Autodesk Inventor part; units mm, degrees
ref_plane "YZ Plane" through (0, 0, 0) normal (1, 0, 0) x (0, 1, 0)
ref_plane "XZ Plane" through (0, 0, 0) normal (0, 1, 0) x (-1, 0, 0)
ref_plane "XY Plane" through (0, 0, 0) normal (0, 0, 1) x (1, 0, 0)
sketch "Sketch1" plane through (0, 0, 0) normal (0, 0, 1) x (1, 0, 0)
  line L0 (3.6662, 6.35) -> (7.3323, 0)
  line L1 (7.3323, 0) -> (3.6662, -6.35)
  line L2 (3.6662, -6.35) -> (-3.6662, -6.35)
  line L3 (-3.6662, -6.35) -> (-7.3323, 0)
  line L4 (-7.3323, 0) -> (-3.6662, 6.35)
  line L5 (-3.6662, 6.35) -> (3.6662, 6.35)
  point P0 (0, 0)
  point P1 (0, 0)
  dimension "d0" = 12.7
extrude "Extrusion1" add sketch "Sketch1" along normal blind 82.55
sketch "Sketch3" plane through (0, 0, 82.55) normal (0, 0, 1) x (1, 0, 0)
  circle A0 centre (0, 0) radius 3.175
  dimension "d4" = 6.35
extrude "Extrusion2" cut sketch "Sketch3" against normal blind 25.4
sketch "Sketch4" plane through (0, 0, 0) normal (0, 0, -1) x (-1, 0, 0)
  circle A0 centre (0, 0) radius 3.175
  dimension "d7" = 6.35
extrude "Extrusion3" cut sketch "Sketch4" against normal blind 25.4
properties part number "WheelAxle" material "Aluminum-6061"
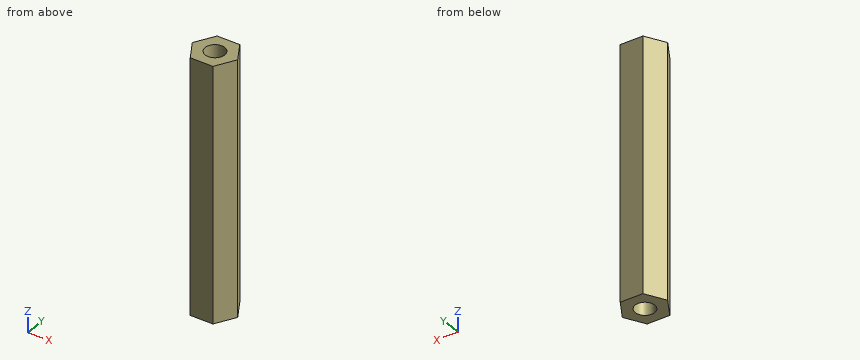
Source: CAD feature listing. Evaluate the final solid. Frame: model axes, mm. Give positions to 0.01 mm unless a question says otherwise; leave off trailing zeros. Write each loop counter-clockwise with the first axis right and the second up, starting at its lowest first coordinate (ties: lowest second). Pieces come first, ordered by that corner, then holes. Notation, with made-up numbers: (10.25, 73) -> (24.25, 73) arc R9 ccw to (24.25, 79) -> close; hole circle Ø8 at (-9, -36.75). An arc over 180 degrees is marked (long way). Return JSON: item names as keys, results as strings. Group by question number.
1. Section A-A, the plane z = 75.5. Output: boundary loops of the cut face in (x, y) (3 decimals).
2. Pin query (flat end, axial travel): pin 1 Ø3 at (x, y) = (-0.5, -0.5) entering from +Z; pin 2 Ø4 at (x, y) = (0, 0) entering from -Z; pin 3 Ø3 at (y, z) = (5, 23.5) entering from -X. Return the tip coordinate at first contact, or that it passes through.
3. Material intervals for line 1 (Y direction, x = 0, z = 73) (3 decimals); line 2 (Y direction, x = -2.5, z = 70.5); line 3 (X direction, y = 1.5, z = 24), sorted ascending. Write a range as from..to.
4. Section C-C, the plane z = 55. Output: boundary loops of the cut face in (x, y).
5. Section B-B, the plane x = 0. Output: boundary loops of the cut face in (y, z) (3 decimals).
6. Section D-D, the plane x = 5.25. Output: boundary loops of the cut face in (y, z), then the cut area to 3 significant figures.
Determined:
{
 "1": {"outline": "(-7.332, 0) -> (-3.666, -6.35) -> (3.666, -6.35) -> (7.332, 0) -> (3.666, 6.35) -> (-3.666, 6.35) -> close; hole circle Ø6.35 at (0, 0)"},
 "2": {"pin 1": "stops at z = 57.15", "pin 2": "stops at z = 25.4", "pin 3": "stops at x = -5.31"},
 "3": {"line 1": "y = -6.35..-3.175, 3.175..6.35", "line 2": "y = -6.35..-1.96, 1.96..6.35", "line 3": "x = -6.47..-2.8, 2.8..6.47"},
 "4": {"outline": "(-7.33, 0) -> (-3.67, -6.35) -> (3.67, -6.35) -> (7.33, 0) -> (3.67, 6.35) -> (-3.67, 6.35) -> close"},
 "5": {"outline": "(-6.35, 0) -> (-3.175, 0) -> (-3.175, 25.4) -> (3.175, 25.4) -> (3.175, 0) -> (6.35, 0) -> (6.35, 82.55) -> (3.175, 82.55) -> (3.175, 57.15) -> (-3.175, 57.15) -> (-3.175, 82.55) -> (-6.35, 82.55) -> close"},
 "6": {"outline": "(-3.61, 0) -> (3.61, 0) -> (3.61, 82.55) -> (-3.61, 82.55) -> close", "area": "595 mm2"}
}
